Can you work these out from the model? Positions are in its coordinate system, mm. A direction names the side the tool comes from. Give positions to 0.01 mm unless a question says otherwise; leave off trailing zeros. Order: outer loops, then holes, each group sorted by start corner. A loop starts at its lowest first (then second) coordinate and runs counter-clockwise, first axis right, second up. Notation, with made-up numbers: (1, 29) - (39, 29) arc R25 cw to (39, 56) - close; hole circle Ø6 at (69, 67.5). An arc over 180 degrees is marked (long way). Write each question's results on one line, items separated by ' | '. Start each with the question number.
from build123d import *

# Parameters (mm, degrees)
F0_R          = 3.96875
F0_R_2        = 2.15265
F1_DEPTH      = 152.4
F3_R          = 2.15265
F4_DEPTH      = 3.175
F4_DEPTH_BACK = 155.575
F5_DEPTH      = 152.4


with BuildPart() as f1:
    # F0 (on Top) → F1 (new body)
    with BuildSketch(Plane.XY):
        Circle(F0_R)
        Circle(F0_R_2, mode=Mode.SUBTRACT)
    extrude(amount=F1_DEPTH)

    # F3 (on face) → F4 (join, two sides)
    with BuildSketch(Plane(origin=(0, 0, 0), x_dir=(1, 0, 0), z_dir=(0, 0, -1))) as f4_sk:
        Polygon((1.984375, -3.4370383213), (3.96875, 0), (1.984375, 3.4370383213), (-1.984375, 3.4370383213), (-3.96875, 0), (-1.984375, -3.4370383213), align=None)
        Circle(F3_R, mode=Mode.SUBTRACT)
    extrude(amount=F4_DEPTH)
    extrude(f4_sk.sketch, amount=-F4_DEPTH_BACK)

    # F5 (cut, through all): a face of the model
    f5_faces = [f1.faces().sort_by_distance(p)[0] for p in [
        (3.1618531236, 1.8254967521, 0),
    ]]
    extrude(f5_faces, amount=-F5_DEPTH, mode=Mode.SUBTRACT)


solid = f1.part
Q1. If we section it at B-B (z = 103): Please give me the cut outline in (x, y), plus the area to 3 significant figures.
Q2. Which directions (+Z, -Z, +X, -X, +Y, -Y) give clear straight access to the entire face, cutting with the end or side of a thin tool? Please do faces 1 (the flat face through (0, 3.437, -2)), 2 (the flat face through (-2.963, -1.743, 153.965)), 3 (the flat face through (2.99, -1.694, 153.965)), 4 (the flat face through (0, 3.437, 154)), 5 (the flat face through (0, -3.437, -2)).
Q3. Will these pins go through, and if not, where does the flat tip stop? P1, Ø3.5, axis at x = 1, z = -2, coming from the +Y side; P2, Ø1, axis at x = -0.5, z = 154.5, coming from the -Y side; P3, Ø3.5, axis at x = -1, z = -1.5, coming from the -Y side.
Q4. If I drill on probe 1 along Y at (x, z) = (0, 100.5); probe 2 along Y at (x, z) = (0, -2.1), over which ranges is the centre line in solid material (lowest first)? Write a range as from..to.
Q5. If we section it at A-A (x = 0): Please give me the cut outline in (y, z) (3 decimals), plus the area to 3 significant figures.
Findings below:
1) outline: (1.98, 3.44) arc R3.97 ccw (long way) to (3.97, 0) - close; hole circle Ø4.31 at (0, 0) | area: 33.5 mm2
2) face 1: -Z, +X, -X, +Y | face 2: +Z, -X, -Y | face 3: +Z, +X, -Y | face 4: +Z, +X, -X, +Y | face 5: -Z, +X, -X, -Y
3) P1: stops at y = 3.44 | P2: stops at y = -3.44 | P3: stops at y = -3.97
4) probe 1: y = -3.97..-2.15, 2.15..3.97 | probe 2: y = -3.44..-2.15, 2.15..3.44
5) outline: (-3.969, 0) - (-3.437, 0) - (-3.437, -3.175) - (-2.153, -3.175) - (-2.153, 155.575) - (-3.437, 155.575) - (-3.437, 152.4) - (-3.969, 152.4) - close; (2.153, -3.175) - (3.437, -3.175) - (3.437, 0) - (3.969, 0) - (3.969, 152.4) - (3.437, 152.4) - (3.437, 155.575) - (2.153, 155.575) - close | area: 570 mm2
